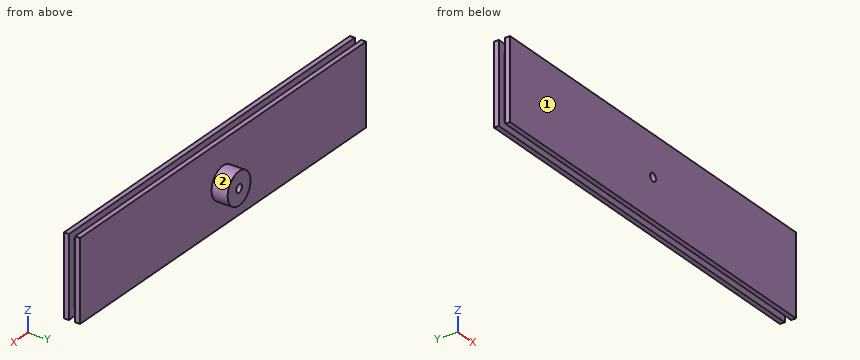
Autodesk Inventor part; units mm, degrees
ref_plane "YZ Plane" through (0, 0, 0) normal (1, 0, 0) x (0, 1, 0)
ref_plane "XZ Plane" through (0, 0, 0) normal (0, 1, 0) x (-1, 0, 0)
ref_plane "XY Plane" through (0, 0, 0) normal (0, 0, 1) x (1, 0, 0)
sketch "Sketch1" plane through (0, 0, 0) normal (0, 1, 0) x (-1, 0, 0)
  line L0 (-125, -25) -> (125, -25)
  line L1 (125, -25) -> (125, 25)
  line L2 (125, 25) -> (-125, 25)
  line L3 (-125, 25) -> (-125, -25)
  line L4 (-125, -25) -> (125, 25) construction
  line L5 (125, -25) -> (-125, 25) construction
  point P0 (0, 0)
  dimension "d0" = 250
  dimension "d1" = 50
extrude "Extrusion1" add sketch "Sketch1" along normal blind 3
sketch "Sketch2" plane through (0, 3, 0) normal (0, 1, 0) x (1, 0, 0)
  line L0 (120, 20) -> (-120, 20)
  line L1 (-120, 20) -> (-120, -20)
  line L2 (-120, -20) -> (120, -20)
  line L3 (120, -20) -> (120, 20)
  line L4 (120, 20) -> (-120, -20) construction
  line L5 (-120, 20) -> (120, -20) construction
  point P0 (0, 0)
  dimension "d4" = 240
  dimension "d5" = 40
extrude "Extrusion2" add sketch "Sketch2" along normal blind 4
sketch "Sketch3" plane through (0, 7, 0) normal (0, 1, 0) x (1, 0, 0)
  line L0 (125, 25) -> (-125, 25)
  line L1 (-125, 25) -> (-125, -25)
  line L2 (-125, -25) -> (125, -25)
  line L3 (125, -25) -> (125, 25)
  line L4 (125, 25) -> (-125, -25) construction
  line L5 (-125, 25) -> (125, -25) construction
  point P0 (0, 0)
extrude "Extrusion3" add sketch "Sketch3" along normal blind 3
sketch "Sketch4" plane through (0, 10, 0) normal (0, 1, 0) x (1, 0, 0)
  circle A0 centre (0, 0) radius 10
  dimension "d10" = 20
extrude "Extrusion4" add sketch "Sketch4" along normal blind 10
sketch "Sketch5" plane through (0, 20, 0) normal (0, 1, 0) x (1, 0, 0)
  circle A0 centre (0, 0) radius 2.5
  dimension "d13" = 5
extrude "Extrusion5" cut sketch "Sketch5" against normal blind 30
properties part number "trail 7" material "Polypropylene"
Build history of the part. All positions in model axes, mm. Face numbers are marked on the shaded views. A direction names the side the tool comes from. Give positions to 0.01 mm unless a question says otherwise; leave off trailing zeros. Loops run counter-clockwise (first coordinate to the right, second up) from the corner with the lowest first, then second, coordinate; pieces in that order, holes last. Notation, with made-up numbers: (62.5, -39) -> (90.5, -39) arc R26 cw to (90.5, -13) -> close; hole circle Ø1 at (83.25, 58.25). An arc over 180 degrees is marked (long way). One line per question, with ' | ' between items.
Q1. Drill centre lines: line 1 along Z through (x, y) = (0, 16); line 2 along X through (y, z) = (4, 0). Where is each one in solid material? Low to high. Write a range as [from, to].
Filled sheet:
line 1: z = [-10, -2.5], [2.5, 10] | line 2: x = [-120, -2.5], [2.5, 120]
Q2. Cut at A-A, the plane x = 0. Write the cut outline in (y, z).
Filled sheet:
outline: (0, -25) -> (3, -25) -> (3, -20) -> (7, -20) -> (7, -25) -> (10, -25) -> (10, -10) -> (20, -10) -> (20, -2.5) -> (0, -2.5) -> close; (0, 2.5) -> (20, 2.5) -> (20, 10) -> (10, 10) -> (10, 25) -> (7, 25) -> (7, 20) -> (3, 20) -> (3, 25) -> (0, 25) -> close
Q3. Drop flat-ended pins along their axis: pin 1 (4 mm diameter, centred on x = 0, z = 0, fed in from -Y); pin 2 (2 mm diameter, centred on x = -11, y = 5, fed in from -Z); pin 3 (2 mm diameter, centred on x = 32, z = -2.5, fed in from +Y); pin 4 (1.2 mm diameter, centred on x = 46.5, y = 4.5, fed in from +Z). Give the stop position or say it passes through.
Filled sheet:
pin 1: passes through | pin 2: stops at z = -20 | pin 3: stops at y = 10 | pin 4: stops at z = 20
Q4. Cut at D-D, the plane x = -40. Write the cut outline in (y, z), plus the area to 3 significant figures.
Filled sheet:
outline: (0, -25) -> (3, -25) -> (3, -20) -> (7, -20) -> (7, -25) -> (10, -25) -> (10, 25) -> (7, 25) -> (7, 20) -> (3, 20) -> (3, 25) -> (0, 25) -> close | area: 460 mm²
Q5. Cut at B-B, the plane z = 0. Write the cut outline in (x, y).
Filled sheet:
outline: (-125, 0) -> (-2.5, 0) -> (-2.5, 20) -> (-10, 20) -> (-10, 10) -> (-125, 10) -> (-125, 7) -> (-120, 7) -> (-120, 3) -> (-125, 3) -> close; (2.5, 0) -> (125, 0) -> (125, 3) -> (120, 3) -> (120, 7) -> (125, 7) -> (125, 10) -> (10, 10) -> (10, 20) -> (2.5, 20) -> close
Q6. Tool access for the marked faces 1 and 2: list every direction of +Z, -Z, +X, -X, +Y, -Y with a clear straight run to the whole face (end or side of a thin tool).
Filled sheet:
face 1: +Z, -Z, +X, -X, -Y | face 2: +Y
Q7. Cut at C-C, the plane y = 15.25. Write the cut outline in (x, z), plus the area to 3 significant figures.
Filled sheet:
outline: circle Ø20 at (0, 0); hole circle Ø5 at (0, 0) | area: 295 mm²
